Input: part model. Units: mm. Frame: model coordinates. Round coordinates to 2 decimals unless told otherwise and drop trailing zeros. Loops run counter-clockwise (first coordinate to the right, second up) from the corner with the lowest first, then second, coordinate; pieces in that order, holes last. Notation, with made-up numbers: (88.25, 18.5) -> (126.25, 18.5) arc R16 ccw to (126.25, 23.5) -> close; hole circle Ø8 at (52.25, 41.5). An arc over 180 degrees is marked (long way). Answer in a Markdown table with one row per item. Add a question column.
Q1. Ray query, L1, parallel to Y at x = 0, z = 1.1; L2, parallel to Y at x = 4, z = 0.9; L3, parallel to Y at x = -3.75, z = 2.4. Return the intervals inside material, ascending. Write a range as from..to.
Q2. Section B-B, the plane z = 0.6. Give the number of separate pieces and of enclosed holes in the cut face, and give its area (3 significant figures).
Q3. Section C-C, the plane x = 0. Output: boundary loops of the cut face in (y, z) (3 decimals), and give its area (3 significant figures).
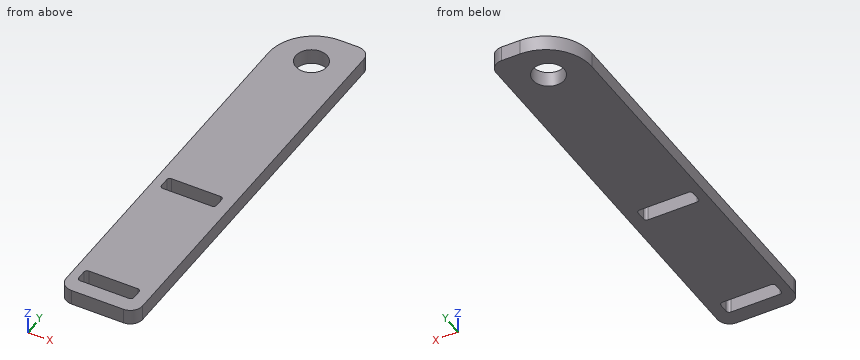
```python
from build123d import *

# Parameters (mm, degrees)
SKETCH1_R           = 3.25
BOSS_EXTRUDE1_DEPTH = 3.175


with BuildPart() as part:
    # Sketch1 → Boss-Extrude1 (new body)
    with BuildSketch(Plane.XY):
        with BuildLine():
            Line((-7.9375, -1.830947062), (-7.9375, -75.490947062))
            ThreePointArc((-7.9375, -75.490947062), (-7.193551224, -77.286998286), (-5.3975, -78.030947062))
            Line((-5.3975, -78.030947062), (5.3975, -78.030947062))
            ThreePointArc((5.3975, -78.030947062), (7.193551224, -77.286998286), (7.9375, -75.490947062))
            Line((7.9375, -75.490947062), (7.9375, 5.154052938))
            ThreePointArc((7.9375, 5.154052938), (7.193551224, 6.950104162), (5.3975, 7.694052938))
            Line((5.3975, 7.694052938), (1.5875, 7.694052938))
            ThreePointArc((1.5875, 7.694052938), (-5.147692091, 4.904245029), (-7.9375, -1.830947062))
        make_face()
        Circle(SKETCH1_R, mode=Mode.SUBTRACT)
        with BuildLine():
            Line((-5.3975, -71.680947062), (4.7625, -71.680947062))
            ThreePointArc((4.7625, -71.680947062), (5.211512806, -71.866934256), (5.3975, -72.315947062))
            Line((5.3975, -72.315947062), (5.3975, -74.220947062))
            ThreePointArc((5.3975, -74.220947062), (5.211512806, -74.669959868), (4.7625, -74.855947062))
            Line((4.7625, -74.855947062), (-5.3975, -74.855947062))
            ThreePointArc((-5.3975, -74.855947062), (-5.846512806, -74.669959868), (-6.0325, -74.220947062))
            Line((-6.0325, -74.220947062), (-6.0325, -72.315947062))
            ThreePointArc((-6.0325, -72.315947062), (-5.846512806, -71.866934256), (-5.3975, -71.680947062))
        make_face(mode=Mode.SUBTRACT)
        with BuildLine():
            Line((-5.3975, -41.518447062), (4.7625, -41.518447062))
            ThreePointArc((4.7625, -41.518447062), (5.211512806, -41.704434256), (5.3975, -42.153447062))
            Line((5.3975, -42.153447062), (5.3975, -44.058447062))
            ThreePointArc((5.3975, -44.058447062), (5.211512806, -44.507459868), (4.7625, -44.693447062))
            Line((4.7625, -44.693447062), (-5.3975, -44.693447062))
            ThreePointArc((-5.3975, -44.693447062), (-5.846512806, -44.507459868), (-6.0325, -44.058447062))
            Line((-6.0325, -44.058447062), (-6.0325, -42.153447062))
            ThreePointArc((-6.0325, -42.153447062), (-5.846512806, -41.704434256), (-5.3975, -41.518447062))
        make_face(mode=Mode.SUBTRACT)
    extrude(amount=BOSS_EXTRUDE1_DEPTH)


solid = part.part
```
Answer block:
| question | item | result |
|---|---|---|
| 1 | L1 | -78.03..-74.86, -71.68..-44.69, -41.52..-3.25, 3.25..7.56 |
| 1 | L2 | -78.03..-74.86, -71.68..-44.69, -41.52..7.69 |
| 1 | L3 | -78.03..-74.86, -71.68..-44.69, -41.52..6.06 |
| 2 | separate pieces | 1 |
| 2 | enclosed holes | 3 |
| 2 | area | 1,230 mm^2 |
| 3 | outline | (-78.031, 0) -> (-74.856, 0) -> (-74.856, 3.175) -> (-78.031, 3.175) -> close; (-71.681, 0) -> (-44.693, 0) -> (-44.693, 3.175) -> (-71.681, 3.175) -> close; (-41.518, 0) -> (-3.25, 0) -> (-3.25, 3.175) -> (-41.518, 3.175) -> close; (3.25, 0) -> (7.561, 0) -> (7.561, 3.175) -> (3.25, 3.175) -> close |
| 3 | area | 231 mm^2 |
